from build123d import *

# Parameters (mm, degrees)
SKETCH1_W                = 13
SKETCH1_H                = 13
BALL_BEARING_BLOCK_DEPTH = 29.5
SKETCH2_W                = 35
SKETCH2_H                = 4
PADDLE_PLATE_DEPTH       = 29.5
SKETCH3_R                = 5.125
BALLBEARING_1_DEPTH      = 5.25
BALLBEARING_START        = -5
SKETCH4_R                = 5.125
BALLBEARING_2_DEPTH      = 5
SKETCH5_R                = 3
ACHSE_DEPTH              = 19.25
FILLET1_R                = 5
FILLET2_R                = 5
FILLET3_R                = 2
FILLET4_R                = 2
FILLET7_R                = 2
SKETCH6_R                = 1.625
M3_PADDLE_SCREWS_DEPTH   = 4
SKETCH8_W                = 22.5
SKETCH8_H                = 29.5
TOP_PLATE_DEPTH          = 1.5
SKETCH7_R                = 6.25
MAGNET_POCKET_DEPTH      = 4.5


with BuildPart() as part:
    # Sketch1 → Ball Bearing Block (new body)
    with BuildSketch(Plane(origin=(0, 0, 0), x_dir=(1, 0, 0), z_dir=(0, 1, 0))):
        Rectangle(SKETCH1_W, SKETCH1_H)
    extrude(amount=BALL_BEARING_BLOCK_DEPTH)

    # Sketch2 → Paddle Plate (add)
    with BuildSketch(Plane.XZ):
        with Locations((-24, 0)):
            Rectangle(SKETCH2_W, SKETCH2_H)
    extrude(amount=-PADDLE_PLATE_DEPTH)

    # Sketch3 → Ballbearing 1 (cut)
    with BuildSketch(Plane(origin=(0, 29.5, 0), x_dir=(1, 0, 0), z_dir=(0, 1, 0))):
        with Locations(Location((0, 0, 0), (0, 0, 270))):
            Circle(SKETCH3_R)
    extrude(amount=-BALLBEARING_1_DEPTH, mode=Mode.SUBTRACT)

    # Sketch4 → Ballbearing 2 (cut)
    with BuildSketch(Plane.XZ.offset(BALLBEARING_START)):
        with Locations(Location((0, 0, 0), (0, 0, 90))):
            Circle(SKETCH4_R)
    extrude(amount=BALLBEARING_2_DEPTH, mode=Mode.SUBTRACT)

    # Sketch5 → Achse (cut)
    with BuildSketch(Plane(origin=(0, 24.25, 0), x_dir=(1, 0, 0), z_dir=(0, 1, 0))):
        with Locations(Location((0, 0, 0), (0, 0, 270))):
            Circle(SKETCH5_R)
    extrude(amount=-ACHSE_DEPTH, mode=Mode.SUBTRACT)

    # Fillet1
    fillet1_edges = [part.edges().sort_by_distance(p)[0] for p in [
        (6.5, 14.75, -6.5),
    ]]
    fillet(fillet1_edges, radius=FILLET1_R)

    # Fillet2
    fillet2_edges = [part.edges().sort_by_distance(p)[0] for p in [
        (6.5, 14.75, 6.5),
    ]]
    fillet(fillet2_edges, radius=FILLET2_R)

    # Fillet3
    fillet3_edges = [part.edges().sort_by_distance(p)[0] for p in [
        (-6.5, 14.75, -6.5),
    ]]
    fillet(fillet3_edges, radius=FILLET3_R)

    # Fillet4
    fillet4_edges = [part.edges().sort_by_distance(p)[0] for p in [
        (-6.5, 14.75, 6.5),
    ]]
    fillet(fillet4_edges, radius=FILLET4_R)

    # Fillet7
    fillet7_edges = [part.edges().sort_by_distance(p)[0] for p in [
        (-6.5, 14.75, 2),
    ]]
    fillet(fillet7_edges, radius=FILLET7_R)

    # Sketch6 → M3 Paddle Screws (cut)
    with BuildSketch(Plane(origin=(0, 0, -2), x_dir=(-1, 0, 0), z_dir=(0, 0, -1))):
        with Locations((36.5, 8.25)):
            Circle(SKETCH6_R)
        with Locations(Location((36.5, 21.25, 0), (0, 0, 180))):
            Circle(SKETCH6_R)
    extrude(amount=-M3_PADDLE_SCREWS_DEPTH, mode=Mode.SUBTRACT)

    # Sketch8 → Top Plate (add)
    with BuildSketch(Plane(origin=(0, 0, -2), x_dir=(-1, 0, 0), z_dir=(0, 0, -1))):
        with Locations((17.75, 14.75)):
            Rectangle(SKETCH8_W, SKETCH8_H)
    extrude(amount=TOP_PLATE_DEPTH)

    # Sketch7 → Magnet Pocket (cut)
    with BuildSketch(Plane(origin=(0, 0, 2), x_dir=(-1, 0, 0), z_dir=(0, 0, -1))):
        with Locations((22, 14.75)):
            Circle(SKETCH7_R)
    extrude(amount=MAGNET_POCKET_DEPTH, mode=Mode.SUBTRACT)


solid = part.part
Here's how the part is built. I have some questions about the finished solid (model axes, mm). A direction names the side the tool comes from. Coordinates: 2 decimals unless noted, no trailing zeros. Order: outer loops, then holes, each group sorted by start corner. A loop starts at its lowest first (then second) coordinate and runs counter-clockwise, first axis right, second up. Notation, with made-up numbers: (-18.5, 14.5) -> (-10.5, 14.5) arc R22 ccw to (-10.5, 29.5) -> close; hole circle Ø6 at (-2, 30.25). An arc over 180 degrees is marked (long way). Answer in a Markdown table with one row per item.
(1) I want a section at A-A on z = 0. List the corners of the cut face in (x, y) for me (3 decimals), then the cut area to 3 significant figures.
Answer key:
| item | result |
|---|---|
| outline | (-41.5, 0) -> (-5.125, 0) -> (-5.125, 5) -> (-3, 5) -> (-3, 24.25) -> (-5.125, 24.25) -> (-5.125, 29.5) -> (-41.5, 29.5) -> close; (3, 5) -> (5.125, 5) -> (5.125, 0) -> (6.5, 0) -> (6.5, 29.5) -> (5.125, 29.5) -> (5.125, 24.25) -> (3, 24.25) -> close; hole circle Ø3.25 at (-36.5, 8.25); hole circle Ø3.25 at (-36.5, 21.25); hole circle Ø12.5 at (-22, 14.75) |
| area | 1,060 mm^2 |
(2) I want a section at C-C on x = -36.5. List the corners of the cut face in (y, z) for me (3 decimals).
Answer key:
| item | result |
|---|---|
| outline | (0, -2) -> (6.625, -2) -> (6.625, 2) -> (0, 2) -> close; (9.875, -2) -> (19.625, -2) -> (19.625, 2) -> (9.875, 2) -> close; (22.875, -2) -> (29.5, -2) -> (29.5, 2) -> (22.875, 2) -> close |
(3) Will these pins go through, and if not, where does the flat tip stop? pin 1 Ø4 at (x, y) = (-37, 19.5) entering from -Z; pin 2 Ø14.5 at (x, y) = (-22, 14.75) entering from -Z; pin 3 Ø4 at (x, y) = (-14.5, 11) entering from +Z.
Answer key:
| item | result |
|---|---|
| pin 1 | z = -2 |
| pin 2 | z = -3.5 |
| pin 3 | z = 2 |
(4) I want a section at B-B on y = 20.25. List the corners of the cut face in (x, z) for me.
Answer key:
| item | result |
|---|---|
| outline | (-41.5, -2) -> (-37.78, -2) -> (-37.78, 2) -> (-41.5, 2) -> close; (-35.22, -2) -> (-29, -2) -> (-29, -3.5) -> (-6.5, -3.5) -> (-6.5, -4.5) arc R2 ccw to (-4.5, -6.5) -> (1.5, -6.5) arc R5 ccw to (6.5, -1.5) -> (6.5, 1.5) arc R5 ccw to (1.5, 6.5) -> (-4.5, 6.5) arc R2 ccw to (-6.5, 4.5) -> (-6.5, 4) arc R2 cw to (-8.5, 2) -> (-19.03, 2) -> (-19.03, -2.5) -> (-24.97, -2.5) -> (-24.97, 2) -> (-35.22, 2) -> close; hole circle Ø6 at (0, 0) |
(5) Please list where these lines run through material, in increasing order: probe 1 along Y at (x, z) = (-36.5, 1.1) (3 decimals); probe 2 along X at (y, z) = (7.25, -1); probe 3 along Z at (x, y) = (-16, 15).
Answer key:
| item | result |
|---|---|
| probe 1 | 0 to 6.625, 9.875 to 19.625, 22.875 to 29.5 |
| probe 2 | -41.5 to -37.78, -35.22 to -2.83, 2.83 to 6.5 |
| probe 3 | -3.5 to -2.5 |
(6) On a 3-axis mill with a long thin cutter (end or side, diameter ignored), from which of +Z, -Z, +X, -X, +Y, -Y can I reach the whole of each face in a straight line? I mean faces 1 (the face through (-5.003, 26.912, -1.111)), 2 (the face through (-5.9, 14.96, 5.93)), 3 (the face through (-35, 15, -2)), 4 (the face through (-0.1, 5, 3.3)). Say none if no direction works.
Answer key:
| item | result |
|---|---|
| face 1 | +Y |
| face 2 | +Z, -X, +Y, -Y |
| face 3 | -Z, -X, +Y, -Y |
| face 4 | -Y |
(7) I want a section at D-D on x = 0. List the corners of the cut face in (y, z) for me (3 decimals).
Answer key:
| item | result |
|---|---|
| outline | (0, -6.5) -> (29.5, -6.5) -> (29.5, -5.125) -> (24.25, -5.125) -> (24.25, -3) -> (5, -3) -> (5, -5.125) -> (0, -5.125) -> close; (0, 5.125) -> (5, 5.125) -> (5, 3) -> (24.25, 3) -> (24.25, 5.125) -> (29.5, 5.125) -> (29.5, 6.5) -> (0, 6.5) -> close |
(8) Thinking about a two-plate mould opening in Z: for faces 5 (the face through (-29, 15, 2)), 6 (the face through (0.1, 24.25, 3.3)), 7 (the face through (-17.39, 18.97, -0.22)), which applies, +Z half, -Z half, draft (parallel to the pull), parting line (faces both ways), or undercut?
Answer key:
| item | result |
|---|---|
| face 5 | +Z half |
| face 6 | undercut |
| face 7 | draft |
